Autodesk Inventor part; units mm, degrees
ref_plane "YZ Plane" through (0, 0, 0) normal (1, 0, 0) x (0, 1, 0)
ref_plane "XZ Plane" through (0, 0, 0) normal (0, 1, 0) x (-1, 0, 0)
ref_plane "XY Plane" through (0, 0, 0) normal (0, 0, 1) x (1, 0, 0)
sketch "スケッチ1" plane through (0, 0, 0) normal (0, 0, 1) x (1, 0, 0)
  line L0 (0, 0) -> (52.6795, 0)
  line L1 (2.6795, -10) -> (52.6795, -10)
  line L2 (52.6795, 0) -> (52.6795, -10)
  line L3 (2.6795, -10) -> (-83.923, -60)
  line L4 (-36.9615, -21.3397) -> (0, 0)
  line L5 (-83.923, -60) -> (-93.923, -42.6795)
  line L6 (-93.923, -42.6795) -> (-85.2628, -37.6795)
  line L7 (-85.2628, -37.6795) -> (-41.9615, -12.6795)
  line L8 (-41.9615, -12.6795) -> (-36.9615, -21.3397)
  line L9 (-88.923, -51.3397) -> (-45.6218, -26.3397)
  line L10 (-45.6218, -26.3397) -> (-40.6218, -35)
  dimension "d1" = 50
  dimension "d2" = 10
  dimension "d3" = 100
  dimension "d4" = 150
  dimension "d5" = 10
  dimension "d6" = 20
  dimension "d42" = 60
  dimension "d43" = 50
  dimension "d44" = 10
extrude "押し出し1" add sketch "スケッチ1" along normal mid plane 5 contours L0 L2 L1 L3 L10 L9 L5 L6 L7 L8 L4
sketch "スケッチ2" plane through (0, 0, 2.5) normal (0, 0, 1) x (1, 0, 0)
  line L0 (46.4795, -7.1) -> (49.6795, -7.1)
  line L1 (49.6795, -7.1) -> (49.6795, -2.9)
  line L2 (49.6795, -2.9) -> (46.4795, -2.9)
  line L3 (46.4795, -2.9) -> (46.4795, -7.1)
  line L4 (46.4795, -7.1) -> (49.6795, -2.9) construction
  line L5 (49.6795, -7.1) -> (46.4795, -2.9) construction
  line L6 (52.6795, 0) -> (0, 0)
  line L7 (2.6795, -10) -> (52.6795, -10)
  line L8 (52.6795, -10) -> (52.6795, 0)
  point P0 (48.0795, -5)
  dimension "d14" = 3
  dimension "d15" = 3.2
  dimension "d64" = 4.2
  dimension "d65" = 2.9
extrude "押し出し2" cut sketch "スケッチ2" against normal blind 5
sketch "スケッチ5" plane through (0, 0, 2.5) normal (0, 0, 1) x (1, 0, 0)
  line L0 (-41.9615, -12.6795) -> (-93.923, -42.6795)
  line L1 (-93.923, -42.6795) -> (-88.923, -51.3397)
  circle A0 centre (-87.0929, -44.5096) radius 3.05
  point P0 (0, 0)
  dimension "d45" = 5
  dimension "d46" = 5
  dimension "d47" = 6.1
hole "穴3" at (-87.0929, -44.5096, 2.5) direction (0, 0, -1) diameter 6.1 end through all
fillet "フィレット2" radius 2 10 edges at (-93.923, -42.6795, 0) (-88.923, -51.3397, 0) (-41.9615, -12.6795, 0) (-36.9615, -21.3397, 0) (-40.6218, -35, 0) (-45.6218, -26.3397, 0) (2.6795, -10, 0) (0, 0, 0) (52.6795, 0, 0) (52.6795, -10, 0)
sketch "スケッチ6" plane through (0, 0, 2.5) normal (0, 0, 1) x (1, 0, 0)
  arc A0 (50.6795, -10) -> (52.6795, -8) centre (50.6795, -8) ccw
  line L0 (52.6795, -8) -> (52.6795, -2)
  arc A1 (52.6795, -2) -> (50.6795, 0) centre (50.6795, -2) ccw
  line L1 (50.6795, 0) -> (0.5359, 0)
  arc A2 (0.5359, 0) -> (-0.4641, -0.2679) centre (0.5359, -2) ccw
  line L2 (-0.4641, -0.2679) -> (-35.2295, -20.3397)
  arc A3 (-37.9615, -19.6077) -> (-35.2295, -20.3397) centre (-36.2295, -18.6077) ccw
  line L3 (-37.9615, -19.6077) -> (-40.9615, -14.4115)
  arc A4 (-40.9615, -14.4115) -> (-43.6936, -13.6795) centre (-42.6936, -15.4115) ccw
  line L4 (-43.6936, -13.6795) -> (-92.191, -41.6795)
  arc A5 (-92.191, -41.6795) -> (-92.923, -44.4115) centre (-91.191, -43.4115) ccw
  line L5 (-92.923, -44.4115) -> (-89.923, -49.6077)
  arc A6 (-89.923, -49.6077) -> (-87.191, -50.3397) centre (-88.191, -48.6077) ccw
  line L6 (-87.191, -50.3397) -> (-47.3538, -27.3397)
  arc A7 (-44.6218, -28.0718) -> (-47.3538, -27.3397) centre (-46.3538, -29.0718) ccw
  line L7 (-44.6218, -28.0718) -> (-41.6218, -33.2679)
  arc A8 (-41.6218, -33.2679) -> (-38.8897, -34) centre (-39.8897, -32.2679) ccw
  line L8 (-38.8897, -34) -> (2.2154, -10.2679)
  arc A9 (3.2154, -10) -> (2.2154, -10.2679) centre (3.2154, -12) ccw
  line L9 (3.2154, -10) -> (50.6795, -10)
  circle A10 centre (-87.0929, -44.5096) radius 3.05
  line L10 (46.4795, -2.9) -> (49.6795, -2.9)
  line L11 (49.6795, -2.9) -> (49.6795, -7.1)
  line L12 (49.6795, -7.1) -> (46.4795, -7.1)
  line L13 (46.4795, -7.1) -> (46.4795, -2.9)
  circle A11 centre (-87.0929, -44.5096) radius 5
  point P0 (0, 0)
  point P1 (-84.5929, -48.8397)
  point P2 (-91.423, -47.0096)
  point P3 (-89.5929, -40.1795)
extrude "押し出し3" cut sketch "スケッチ6" against normal blind 10 contours L6 A6 L5 A11 | L5 A5 L4 A11
sketch "スケッチ7" plane through (0, 0, 2.5) normal (0, 0, 1) x (1, 0, 0)
  line L0 (-43.6936, -13.6795) -> (-89.5929, -40.1795)
  line L1 (-37.9615, -19.6077) -> (-40.9615, -14.4115)
  line L2 (-38.8897, -34) -> (2.2154, -10.2679)
  line L3 (-44.6218, -28.0718) -> (-41.6218, -33.2679)
  circle A0 centre (-43.7917, -19.5096) radius 5
  circle A1 centre (-38.7917, -28.1699) radius 5
  line L4 (46.4795, -2.9) -> (49.6795, -2.9)
  line L5 (49.6795, -2.9) -> (49.6795, -7.1)
  line L6 (49.6795, -7.1) -> (46.4795, -7.1)
  line L7 (46.4795, -7.1) -> (46.4795, -2.9)
  circle A2 centre (-87.0929, -44.5096) radius 3.05
  arc A3 (-89.5929, -40.1795) -> (-84.5929, -48.8397) centre (-87.0929, -44.5096) ccw
  line L8 (-84.5929, -48.8397) -> (-47.3538, -27.3397)
  arc A4 (-44.6218, -28.0718) -> (-47.3538, -27.3397) centre (-46.3538, -29.0718) ccw
  line L9 (-44.6218, -28.0718) -> (-41.6218, -33.2679)
  arc A5 (-41.6218, -33.2679) -> (-38.8897, -34) centre (-39.8897, -32.2679) ccw
  line L10 (-38.8897, -34) -> (2.2154, -10.2679)
  arc A6 (3.2154, -10) -> (2.2154, -10.2679) centre (3.2154, -12) ccw
  line L11 (3.2154, -10) -> (50.6795, -10)
  arc A7 (50.6795, -10) -> (52.6795, -8) centre (50.6795, -8) ccw
  line L12 (52.6795, -8) -> (52.6795, -2)
  arc A8 (52.6795, -2) -> (50.6795, 0) centre (50.6795, -2) ccw
  line L13 (50.6795, 0) -> (0.5359, 0)
  arc A9 (0.5359, 0) -> (-0.4641, -0.2679) centre (0.5359, -2) ccw
  line L14 (-0.4641, -0.2679) -> (-35.2295, -20.3397)
  arc A10 (-37.9615, -19.6077) -> (-35.2295, -20.3397) centre (-36.2295, -18.6077) ccw
  line L15 (-37.9615, -19.6077) -> (-40.9615, -14.4115)
  arc A11 (-40.9615, -14.4115) -> (-43.6936, -13.6795) centre (-42.6936, -15.4115) ccw
  line L16 (-43.6936, -13.6795) -> (-89.5929, -40.1795)
  point P0 (0, 0)
  point P1 (-36.2917, -32.5)
  point P2 (-43.1218, -30.6699)
  point P3 (-46.2917, -15.1795)
  point P4 (-39.4615, -17.0096)
  dimension "d58" = 5
  dimension "d59" = 5
  dimension "d60" = 5
  dimension "d61" = 5
extrude "押し出し4" cut sketch "スケッチ7" against normal blind 10 contours A11 L1 A0 L0 | A1 L2 A5 L3
properties part number "茎固定パーツ"
Model file for the job. Use its own axes, mm. A direction names the side the tool comes from. Round coordinates to 2 decimals unless told otherwise and drop trailing zeros. Order: outer loops, then holes, each group sorted by start corner. A loop starts at its lowest first (then second) coordinate and runs counter-clockwise, first axis right, second up. Notation, with made-up numbers: M 48.25,34.25 L 69.25,34.25 A13 ccw 69.25,42.25 Z; hole C 34.25,33 d1. An arc over 180 degrees is marked long. Write each question's results on one line, items separated by ' | '. Start each with the question number.
(1) Probe probe 1 along Y at (x, z) = (38.5, -2); probe 2 along X at (y, z) = (-19.5, -2); probe 3 along X at (y, z) = (-29, -0.65). List the from-to ranges inside material, lowest first. Write a range as from..to.
(2) Saw through at A-A, the plane y = -5.5. Give the cut face in (x, z).
(3) Saw through at B-B, the plane x = 15. Give the cut face in (y, z), then the cut area to 3 significant figures.
(4) Saw through at C-C, the plane z = 1.25. Give the cut face in (x, y).
(5) Drop flat-ended pins along their axis: pin 1 (1.3 mm diameter, centred on y = -5.5, z = 0, fed in from -X); pin 2 (1.5 mm diameter, centred on x = -40, z = 0.5, fed in from +Y); pin 3 (10 mm diameter, centred on x = -87.09, y = -44.51, fed in from -Z); pin 4 (1 mm diameter, centred on y = -43.5, z = 1.5, fed in from -X). Give the stop position or say it passes through.
(6) Two-plate mould, pull along Y, no slides. Class faces 1 (the face through (27, -10, 0)), 2 (the face through (-87.227, -41.463, -0.035)), 3 (the face through (25, 0, 0)): pulls with the +Y half, pulls with the -Y half, needs draft (parallel to the pull), parting line crosses it, or undercut.
(7) Saw through at D-D, the plane y = -11.5. Give the cut face in (x, z), then the cut area to 3 significant figures.
(8) Which spindle directions (+Z, -Z, +X, -X, +Y, -Y) get a long thin tool onto all of the face, cutting with end or side? Do faces 4 (the face through (-43.882, -29.353, -0.035)), 5 (the face through (-18.09, -10.444, -0.035)), 6 (the face through (46.48, -5, 0)). Say none if no direction does.
Established:
1) probe 1: y = -10..0 | probe 2: x = -53.77..-38.02, -33.78..-13.77 | probe 3: x = -70.23..-50.23, -44.09..-30.23
2) outline: M -9.53,-2.5 L 46.48,-2.5 L 46.48,2.5 L -9.53,2.5 Z; M 49.68,-2.5 L 52.68,-2.5 L 52.68,2.5 L 49.68,2.5 Z
3) outline: M -10,-2.5 L 0,-2.5 L 0,2.5 L -10,2.5 Z | area: 50.0 mm^2
4) outline: M -89.59,-40.18 A5 ccw -84.59,-48.84 L -47.35,-27.34 A2 cw -44.62,-28.07 L -43.12,-30.67 A5 ccw -36.29,-32.5 L 2.22,-10.27 A2 cw 3.22,-10 L 50.68,-10 A2 ccw 52.68,-8 L 52.68,-2 A2 ccw 50.68,0 L 0.54,0 A2 ccw -0.46,-0.27 L -35.23,-20.34 A2 cw -37.96,-19.61 L -39.46,-17.01 A5 ccw -46.29,-15.18 L -85.26,-37.68 Z; hole C -87.09,-44.51 d6.1; hole M 46.48,-7.1 L 49.68,-7.1 L 49.68,-2.9 L 46.48,-2.9 Z
5) pin 1: stops at x = -10.65 | pin 2: stops at y = -15.54 | pin 3: stops at z = -2.5 | pin 4: stops at x = -92.07
6) face 1: pulls with the -Y half | face 2: undercut | face 3: pulls with the +Y half
7) outline: M -19.92,-2.5 L 0.08,-2.5 L 0.08,2.5 L -19.92,2.5 Z | area: 100 mm^2
8) face 4: +Z, -Z, -Y | face 5: +Z, -Z, +Y | face 6: +Z, -Z
